Part model, mm, in its own coordinate system. Round coordinates to 2 decimals unless told otherwise and drop trailing zeros. Write each loop counter-clockwise with the first axis right and the second up, starting at its lowest first coordinate (ties: lowest second). Pieces come first, ordered by that corner, then holes. Notation, with made-up numbers: M 51.5,-40 L 68.5,-40 A28 ccw 68.5,-4 Z; hole C 42.25,-4 d1. An arc over 180 degrees is marked long. Use a Markdown table: item, result. Add a question column.
1) Slice it at A-A on y = 10. Write the cut outline in (x, z).
2) Wall check: probe 1 along Y at (x, z) = (90, 1.9); probe 2 along Y at (x, z) = (7, 0.6); probe 3 along X at (y, z) = (-138.5, 0.7). Give the ranges that are in metal, low to high.
3) Slice it at B-B on x = 90. Write the cut outline in (y, z).
```python
from build123d import *

# Parameters (mm, degrees)
F0_W     = 100
F0_H     = 126
F0_H_2   = 20
F0_R     = 3.9
F1_DEPTH = 4


with BuildPart() as f1:
    # F0 (on Top) → F1 (new body)
    with BuildSketch(Plane.XY):
        with Locations((50, -63)):
            Rectangle(F0_W, F0_H)
        with Locations((50, 10)):
            Rectangle(F0_W, F0_H_2)
        with Locations((10, 10)):
            Circle(F0_R, mode=Mode.SUBTRACT)
        with Locations((90, 10)):
            Circle(F0_R, mode=Mode.SUBTRACT)
        with Locations((50, -136)):
            Rectangle(F0_W, F0_H_2)
        with Locations((10, -136)):
            Circle(F0_R, mode=Mode.SUBTRACT)
        with Locations((90, -136)):
            Circle(F0_R, mode=Mode.SUBTRACT)
    extrude(amount=F1_DEPTH)


solid = f1.part
```
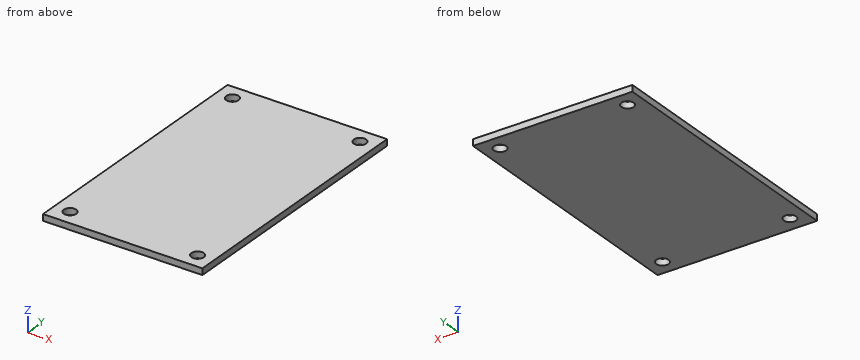
Entries:
| question | item | result |
|---|---|---|
| 1 | outline | M 0,0 L 6.1,0 L 6.1,4 L 0,4 Z; M 13.9,0 L 86.1,0 L 86.1,4 L 13.9,4 Z; M 93.9,0 L 100,0 L 100,4 L 93.9,4 Z |
| 2 | probe 1 | y = -146 to -139.9, -132.1 to 6.1, 13.9 to 20 |
| 2 | probe 2 | y = -146 to -138.49, -133.51 to 7.51, 12.49 to 20 |
| 2 | probe 3 | x = 0 to 7.01, 12.99 to 87.01, 92.99 to 100 |
| 3 | outline | M -146,0 L -139.9,0 L -139.9,4 L -146,4 Z; M -132.1,0 L 6.1,0 L 6.1,4 L -132.1,4 Z; M 13.9,0 L 20,0 L 20,4 L 13.9,4 Z |
